Could you check a few things on this model? Use its own coordinates, in mm. A direction names the side the tool comes from. Coordinates: 2 decimals unless noted, no trailing zeros. Order: outer loops, then holes, each group sorted by start corner. A loop starts at its lowest first (then second) coordinate and runs counter-clockwise, first axis right, second up. Notation, with made-up numbers: (64.25, 2) - (121.25, 2) arc R8 cw to (121.25, 17) - close; hole circle Ø6 at (-8.5, 78.25). An arc over 180 degrees is marked (long way). Answer as a JSON object with one key per item and string values. Group by question number.
(1) Imagine slicing it at D-D, the plane z = -32.5. Write out the boundary of the cut face in (x, y).
(2) Which directions (+Z, -Z, +X, -X, +Y, -Y) give clear straight access to the entire face, cutting with the end or side of a thin tool? Please do faces 1 (the cylindrical face through (22.92, -0.22, -10.2)), 2 (the cylindrical face through (47, 20, 2)), 3 (the cylindrical face through (83, 17, 3)), 4 (the flat face through (94, 19.4, 7.9)), 5 (the flat face through (9, 0, -11)).
(3) Imagine slicing it at A-A, the plane x = 80. Give the number of separate pieces and of enclosed holes in the cut face, and give its area (3 significant figures).
(4) Please list where these lines run through material, in increasing order: probe 1 along Z at (x, y) = (80, 18); probe 2 along Y at (x, z) = (83, 2); probe 3 along Z at (x, y) = (80, -15).
(5) Will these pins go through, and if not, where does the flat tip stop? P1, Ø9.5, axis at x = 11, y = -6, coming from the -Z side; P2, Ø2.5, axis at y = 19.5, z = 7, coming from the -X side; P3, Ø2, axis at x = 80, y = -20, coming from the -Z side.
(6) Imagine slicing it at C-C, the plane x = 39. Write out the boundary of the cut face in (y, z), and give its area (3 significant figures).
(7) Imagine slicing it at B-B, the plane y = 0. Write out the boundary of the cut face in (x, z).
(8) We'd pull the mould along Y, two halves only. Please class faces 6 (the cylindrical face through (49.505, -0.224, -43.298)), 7 (the flat face through (69, -21, 6)), 8 (the flat face through (79, 14, 1)): pulls with the +Y half, pulls with the -Y half, needs draft (parallel to the pull), parting line crosses it, or undercut.
from build123d import *

# Parameters (mm, degrees)
F1_DEPTH  = 16
F2_W      = 70
F2_H      = 3
F3_DEPTH  = 2
F4_W      = 50
F4_H      = 14
F5_DEPTH  = 2
F6_R      = 1
F9_DEPTH  = 2
F11_DEPTH = 42.001
F13_D     = 4
F14_R     = 3
F14_R_2   = 2
F15_DEPTH = 5
F16_R     = 3


# Not quite as in the source:
# - a pattern or mirror of a feature is missing from the dataset's text; its kind, count and spacing are read off the source's solid


with BuildPart() as f1:
    # F0 (on Front) → F1 (new body)
    with BuildSketch(Plane.XZ):
        with BuildLine():
            Line((94, 11), (0, 11))
            ThreePointArc((0, 11), (-11, 0), (0, -11))
            Line((0, -11), (19, -11))
            ThreePointArc((19, -11), (21.7681124643, -11.8361612201), (23.6103896104, -14.064978646))
            ThreePointArc((23.6103896104, -14.064978646), (47.9882051962, -44.6729645648), (84.7744660979, -58.0107943585))
            ThreePointArc((84.7744660979, -58.0107943585), (91.6454906811, -58.677418602), (97.362645896, -62.5464627931))
            Line((97.362645896, -62.5464627931), (98.6602822553, -61))
            ThreePointArc((98.6602822553, -61), (92.2959119196, -56.7859373435), (84.7034264019, -56))
            ThreePointArc((84.7034264019, -56), (49.0672193413, -42.9854179344), (25.4545454545, -13.2909701044))
            ThreePointArc((25.4545454545, -13.2909701044), (22.87535745, -10.1706257081), (19, -9))
            Line((19, -9), (0, -9))
            ThreePointArc((0, -9), (-9, 0), (0, 9))
            Line((0, 9), (94, 9))
            Line((94, 9), (94, 11))
        make_face()
    extrude(amount=F1_DEPTH)

    # F2 (on face) → F3 (join)
    with BuildSketch(Plane.XY.offset(11)):
        with Locations((59, -17.5)):
            Rectangle(F2_W, F2_H)
    extrude(amount=-F3_DEPTH)

    # F4 (on face) → F5 (join)
    with BuildSketch(Plane.XZ.offset(19)):
        with Locations((69, 4)):
            Rectangle(F4_W, F4_H)
    extrude(amount=F5_DEPTH)

    # F6
    f6_edges = [f1.edges().sort_by_distance(p)[0] for p in [
        (69, -21, 11),
        (34, -19, 11),
    ]]
    fillet(f6_edges, radius=F6_R)

    # F7: F1 across plane


with BuildPart() as f1_1:
    add(f1.part)
    add(f1.part.mirror(Plane.XZ))

    # F8 (on face) → F9 (cut)
    with BuildSketch(Plane.XY.offset(11)):
        with BuildLine():
            Line((94, 11.9996714485), (34.088798243, 11.9996714485))
            ThreePointArc((34.088798243, 11.9996714485), (22.0000004897, -0.003428249), (34.0956545385, -11.9996187527))
            Line((34.0956545385, -11.9996187527), (94, -11.9996187527))
            Line((94, -11.9996187527), (94, 11.9996714485))
        make_face()
    extrude(amount=-F9_DEPTH, mode=Mode.SUBTRACT)

    # F10 (on face) → F11 (cut, through all)
    with BuildSketch(Plane.XZ.offset(21)):
        with BuildLine():
            ThreePointArc((50, 5), (47, 2), (50, -1))
            Line((50, -1), (70, -1))
            ThreePointArc((70, -1), (73, 2), (70, 5))
            Line((70, 5), (50, 5))
        make_face()
    extrude(amount=-F11_DEPTH, mode=Mode.SUBTRACT)

    # F13 (through all)
    with Locations(Plane.XZ.offset(21)):
        with Locations((80, 3)):
            Hole(F13_D / 2)

    # F14 (on face) → F15 (join)
    with BuildSketch(Plane(origin=(0, -19, 0), x_dir=(-1, 0, 0), z_dir=(0, 1, 0))):
        with Locations((-80, 3)):
            Circle(F14_R)
        with Locations((-80, 3)):
            Circle(F14_R_2, mode=Mode.SUBTRACT)
    f15 = extrude(amount=F15_DEPTH)

    # F15_copies: F15 across plane
    add(f15.mirror(Plane.ZX))

    # F16
    f16_edges = [f1_1.edges().sort_by_distance(p)[0] for p in [
        (44, 20, -3),
        (94, 20, -3),
        (94, -20, -3),
        (44, -20, -3),
    ]]
    fillet(f16_edges, radius=F16_R)


solid = f1_1.part
Result set:
{
 "1": {"outline": "(34.86, -16) - (37.5, -16) - (37.5, 16) - (34.86, 16) - close"},
 "2": {"face 1": "+X, +Y, -Y", "face 2": "+Y, -Y", "face 3": "none", "face 4": "+Z, +X, +Y, -Y", "face 5": "-Z, -X, +Y, -Y"},
 "3": {"separate pieces": "5", "enclosed holes": "0", "area": "152 mm^2"},
 "4": {"probe 1": "z = 0 to 1, 5 to 6, 9 to 11", "probe 2": "y = -21 to -19, 19 to 21", "probe 3": "z = -57.5 to -55.48, 0 to 1, 5 to 6, 9 to 11"},
 "5": {"P1": "stops at z = -11", "P2": "stops at x = 44", "P3": "stops at z = -3"},
 "6": {"outline": "(-19, 9) - (-12, 9) - (-12, 11) - (-18, 11) arc R1 ccw to (-19, 10) - close; (-16, -37.02) - (16, -37.02) - (16, -34.15) - (-16, -34.15) - close; (12, 9) - (19, 9) - (19, 10) arc R1 ccw to (18, 11) - (12, 11) - close", "area": "120 mm^2"},
 "7": {"outline": "(0, -11) - (19, -11) arc R5 cw to (23.61, -14.06) arc R72 ccw to (84.77, -58.01) arc R14 cw to (97.36, -62.55) - (98.66, -61) arc R16 ccw to (84.7, -56) arc R70 cw to (25.45, -13.29) arc R7 ccw to (19, -9) - (0, -9) arc R9 cw to (0, 9) - (22, 9) - (22, 11) - (0, 11) arc R11 ccw to start"},
 "8": {"face 6": "needs draft", "face 7": "pulls with the -Y half", "face 8": "undercut"}
}
